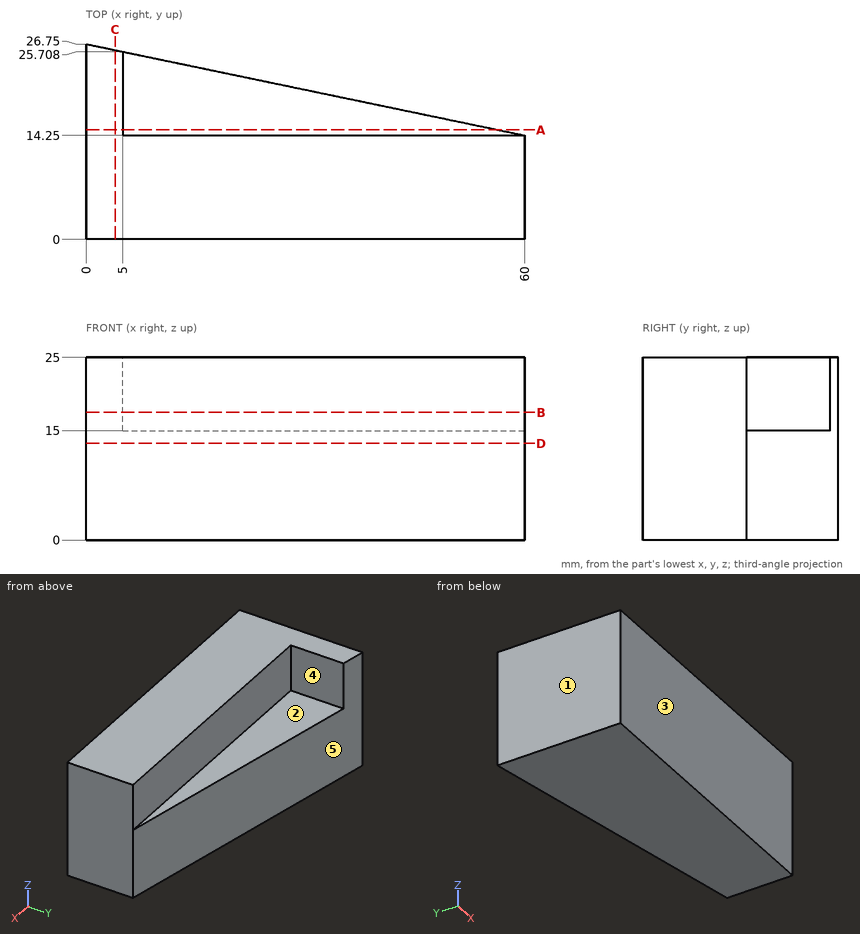
Geometry check sheet. Reference: drawing and pictorial views, mm from the part's lowest x, y, z. A direction names the side the tool comes from. Round coordinates to 2 decimals unless told otherwise and drop trailing zeros. Order: outer loops, then holes, each group sorted by start corner. A loop starts at its lowest first (then second) coordinate and runs counter-clockwise, first axis right, second up. Notation, with made-up numbers: (59.25, -10) - (105.25, -10) arc R16 cw to (105.25, 19) - close; hole circle Ø11 at (-18, -26.75). An arc over 180 degrees is marked (long way). Use a Markdown table: item, result. Add a question column.
1) Gauge pin test, flat ends, axial feed: P1, Ø3, axis at x = 32, z = 10, coming from the +Y side; P2, Ø2, axis at x = 24, z = 9, coming from the +Y side; P3, Ø8, axis at y = 19.5, z = 22.5, coming from the +X side. Record the tip position at first contact, or that the pin passes through.
2) Set-up check for the marked faces 1 and 2: record each of +Z, -Z, +X, -X, +Y, -Y from which the full face is reachable in a straight line by a thin tool's end or side.
3) Mould release check, pull along Y, two halves, no side actions. Record for the marked faces 3, 4 and 5: released by +Y, released by -Y, zero draft, split by the parting line, or undercut.
4) Thickness scan on line 1 along Y through (x, z) = (21, 21); line 2 along Z through (x, y) = (48, 15.5); line 3 along X through (y, z) = (14.75, 18.5). Record the ranges inside material, lowest first.
5) Section check B-B (z = 17.5). Record the cut outline in (x, y).
6) Section check C-C (x = 4). Record the cut outline in (y, z).
7) Section check A-A (y = 15). Record the cut outline in (x, z), then the cut area to 3 significant figures.
8) Section check D-D (z = 13.25). Record the cut outline in (x, y).
Established:
| question | item | result |
|---|---|---|
| 1 | P1 | y = 20.4 |
| 1 | P2 | y = 21.96 |
| 1 | P3 | x = 5 |
| 2 | face 1 | +Z, -Z, -X, +Y, -Y |
| 2 | face 2 | +Z, +X, +Y |
| 3 | face 3 | released by -Y |
| 3 | face 4 | zero draft |
| 3 | face 5 | released by +Y |
| 4 | line 1 | 0 to 14.25 |
| 4 | line 2 | 0 to 15 |
| 4 | line 3 | 0 to 5 |
| 5 | outline | (0, 0) - (60, 0) - (60, 14.25) - (5, 14.25) - (5, 25.71) - (0, 26.75) - close |
| 6 | outline | (0, 0) - (25.92, 0) - (25.92, 25) - (0, 25) - close |
| 7 | outline | (0, 0) - (56.4, 0) - (56.4, 15) - (5, 15) - (5, 25) - (0, 25) - close |
| 7 | area | 896 mm2 |
| 8 | outline | (0, 0) - (60, 0) - (60, 14.25) - (0, 26.75) - close |
